For this review, use the dimensioned drawing (mm, ordinates from the lowest corner) and the shaded views. Round coordinates to 2 decimals unless told otherwise and drop trailing zeros. Write each loop counter-clockwise with the first axis right and the second up, starting at its lowest first coordinate (ties: lowest second). Pieces come first, ordered by that corner, then holes.
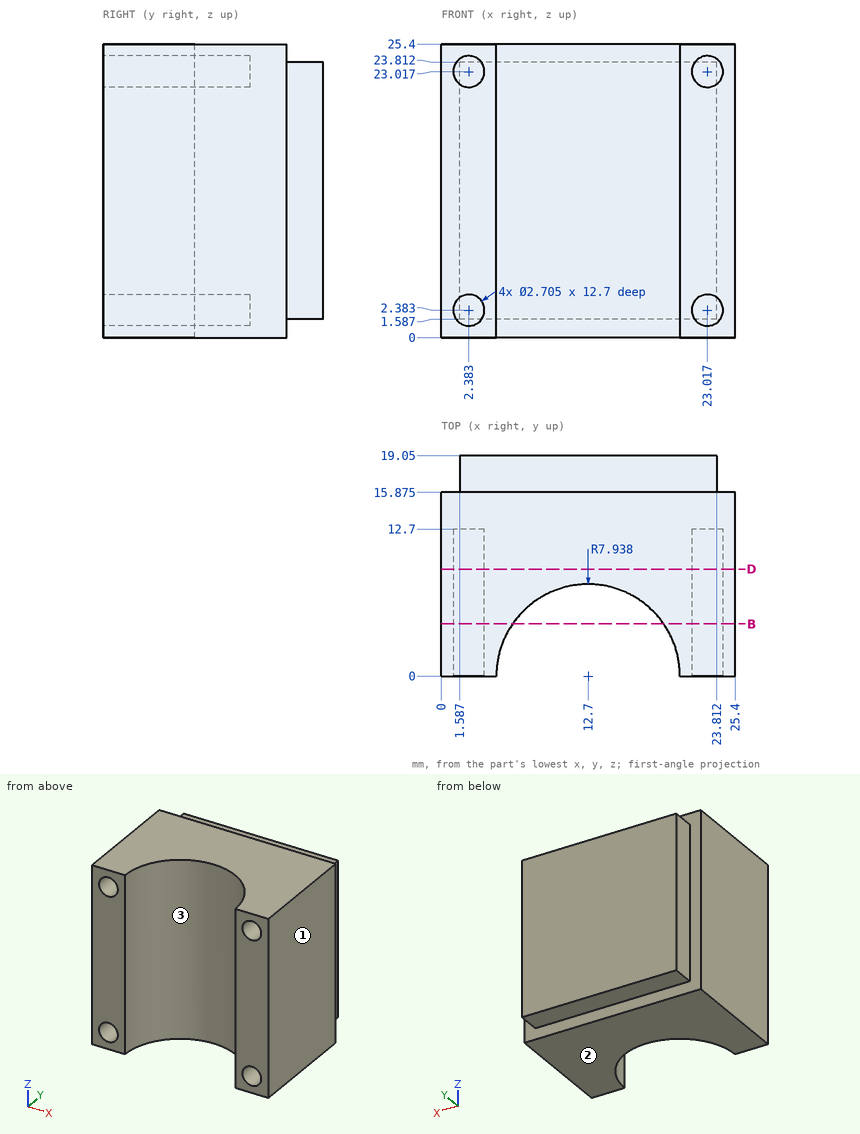
(1) Mouldability with a two-part tool opening along X and no side actions: class the marked faces 1, 2 and 3 as pulls with the +X half, pulls with the -X half, needs draft (parallel to the pull), parting line crosses it, or undercut.
Geometry check:
face 1: pulls with the +X half
face 2: needs draft
face 3: undercut
(2) We need section B-B, the plane y = 4.5. Give the boundary of the cut face in (x, z) (1 decimal), and give its area (3 significant figures).
Geometry check:
outline: (0, 0) - (6.2, 0) - (6.2, 25.4) - (0, 25.4) - close; (19.2, 0) - (25.4, 0) - (25.4, 25.4) - (19.2, 25.4) - close; hole circle Ø2.7 at (2.4, 2.4); hole circle Ø2.7 at (2.4, 23); hole circle Ø2.7 at (23, 2.4); hole circle Ø2.7 at (23, 23)
area: 290 mm2
(3) For line 1 along X through (y, z) = (16.5, 18.75); line 2 along X through (y, z) = (4.5, 5.25), list the stretches that pass through material, from the lowest coordinate up.
Geometry check:
line 1: x = 1.59 to 23.81
line 2: x = 0 to 6.16, 19.24 to 25.4
(4) We need section D-D, the plane y = 9.25. Give the boundary of the cut face in (x, z) (1 decimal), and give its area (3 significant figures).
Geometry check:
outline: (0, 0) - (25.4, 0) - (25.4, 25.4) - (0, 25.4) - close; hole circle Ø2.7 at (2.4, 2.4); hole circle Ø2.7 at (2.4, 23); hole circle Ø2.7 at (23, 2.4); hole circle Ø2.7 at (23, 23)
area: 622 mm2
(5) For pin 1 Ø0.8 at (x, z) = (22.5, 2.5) entering from -Y; pin 2 Ø4 at (x, z) = (8.5, 10) entering from -Y (1 decimal); pin 3 Ø1 at (x, y) = (10.5, 18) entering from -Z, all flat-tipped, find the tip position at first contact; note any pin that passes through.
Geometry check:
pin 1: stops at y = 12.7
pin 2: stops at y = 5
pin 3: stops at z = 1.59
